Verification items for the finished model (mm, model axes). A direction names the side the tool comes from. Coordinates: 2 decimals unless noted, no trailing zeros. Order: outer loops, then holes, each group sorted by start corner. A loop starts at its lowest first (then second) coordinate and runs counter-clockwise, first axis right, second up. Notation, with made-up numbers: (-6.5, 60) -> (30.5, 60) arc R26 ccw to (30.5, 89) -> close; hole circle Ø1 at (74.5, -4). An arc over 180 degrees is marked (long way). Answer as CSV lines item,"result".
```python
from build123d import *

# Parameters (mm, degrees)
SZKIC1_R                    = 14
DODANIE_WYCI_GNI_CIE1_DEPTH = 4.5
SFAZOWANIE2_SIZE2           = 4.345599487
SFAZOWANIE2_SIZE            = 4.5
DODANIE_WYCI_GNI_CIE5_DEPTH = 12
WYTNIJ_WYCI_GNI_CIE2_DEPTH  = 8
SFAZOWANIE4_SIZE            = 4.5
SFAZOWANIE4_SIZE2           = 4.95
ZAOKR_GLENIE2_R             = 0.5
ZAOKR_GLENIE3_R             = 10.5
WYTNIJ_WYCI_GNI_CIE3_DEPTH  = 6


# Some blends are built 0.0001 mm under size
with BuildPart() as part:
    # Szkic1 → Dodanie-wyciągnięcie1 (new body)
    with BuildSketch(Plane.XY):
        Circle(SZKIC1_R)
    extrude(amount=DODANIE_WYCI_GNI_CIE1_DEPTH)

    # Sfazowanie2
    sfazowanie2_edges = [part.edges().sort_by_distance(p)[0] for p in [
        (-14, 0, 4.5),
    ]]
    sfazowanie2_side = [part.faces().sort_by_distance(p)[0] for p in [
        (-14, 0, 4.41308801),
    ]]
    chamfer(sfazowanie2_edges, length=SFAZOWANIE2_SIZE - 0.0001, length2=SFAZOWANIE2_SIZE2 - 0.0001, reference=sfazowanie2_side[0])  # a hair under: the kernel refuses the full size

    # Szkic2 → Dodanie-wyciągnięcie5 (add)
    with BuildSketch(Plane.XY.offset(4.5)):
        with BuildLine():
            Line((9.452124483, 1.965907434), (-0.429502914, 3.5))
            Line((-0.429502914, 3.5), (-8.99763576, 3.5))
            ThreePointArc((-8.99763576, 3.5), (-9.786966842, 0), (-8.99763576, -3.5))
            Line((-8.99763576, -3.5), (-0.429502914, -3.5))
            Line((-0.429502914, -3.5), (9.452124483, -1.965907434))
            ThreePointArc((9.452124483, -1.965907434), (9.654400513, 0), (9.452124483, 1.965907434))
        make_face()
    extrude(amount=DODANIE_WYCI_GNI_CIE5_DEPTH)

    # Szkic8 → Wytnij-wyciągnięcie2 (cut)
    with BuildSketch(Plane(origin=(0, 0, 0), x_dir=(-1, 0, 0), z_dir=(0, 0, -1))):
        with BuildLine():
            Line((-9.452124483, 1.965907434), (-13.654313406, 3.091880562))
            ThreePointArc((-13.654313406, 3.091880562), (-14.042737349, 0), (-13.654313406, -3.091880562))
            Line((-13.654313406, -3.091880562), (-9.452124483, -1.965907434))
            ThreePointArc((-9.452124483, -1.965907434), (-9.654400513, 0), (-9.452124483, 1.965907434))
        make_face()
    extrude(amount=-WYTNIJ_WYCI_GNI_CIE2_DEPTH, mode=Mode.SUBTRACT)

    # Sfazowanie4
    sfazowanie4_edges = [part.edges().sort_by_distance(p)[0] for p in [
        (9.654400513, 0, 16.5),
    ]]
    sfazowanie4_side = [part.faces().sort_by_distance(p)[0] for p in [
        (9.654400513, 0, 8.25),
    ]]
    chamfer(sfazowanie4_edges, length=SFAZOWANIE4_SIZE, length2=SFAZOWANIE4_SIZE2, reference=sfazowanie4_side[0])

    # Zaokrąglenie2
    zaokr_glenie2_edges = [part.edges().sort_by_distance(p)[0] for p in [
        (-9.786966842, 0, 16.5),
        (-4.713569337, -3.5, 16.5),
        (1.655695985, -3.17627922, 16.5),
        (-4.713569337, 3.5, 16.5),
        (1.655695985, 3.17627922, 16.5),
        (4.704400513, 0, 16.5),
        (6.663505686, 2.398832011, 14.338418901),
        (9.654400513, 0, 12),
        (6.663505686, -2.398832011, 14.338418901),
    ]]
    fillet(zaokr_glenie2_edges, radius=ZAOKR_GLENIE2_R)

    # Zaokrąglenie3
    # the kernel refuses this fillet: 10.5 mm, written as the material it takes off along each edge
    with BuildSketch(Plane(origin=(-1.239696749, -7, 16.5), x_dir=(0.15340925660527832, 0.9881627396273429, 0), z_dir=(0.9881627396273429, -0.15340925660527832, 0))) as zaokr_glenie3_piece_1:
        with BuildLine():
            CenterArc((10, -0.5), 0.5, 0, 90)
            Line((10.5, -0.5), (10.5, 0))
            Line((10.5, 0), (10, 0))
        make_face()
    revolve(axis=Axis((-1.239696749, -7, 16.5), (0, 0, 1)), revolution_arc=8.824549996, mode=Mode.SUBTRACT)
    with BuildSketch(Plane(origin=(-1.239696749, 7, 16.5), x_dir=(0, -1, 0), z_dir=(-1, 0, 0))) as zaokr_glenie3_piece_2:
        with BuildLine():
            CenterArc((10, -0.5), 0.5, 0, 90)
            Line((10.5, -0.5), (10.5, 0))
            Line((10.5, 0), (10, 0))
        make_face()
    revolve(axis=Axis((-1.239696749, 7, 16.5), (0, 0, 1)), revolution_arc=8.824549996, mode=Mode.SUBTRACT)
    with BuildSketch(Plane(origin=(-0.429502914, -3.5, 4.5), x_dir=(0.9881627396273429, 0.15340925660527846, 0), z_dir=(0, 0, 1))) as zaokr_glenie3_piece_3:
        with BuildLine():
            CenterArc((ZAOKR_GLENIE3_R * 0.0771613176062, ZAOKR_GLENIE3_R), ZAOKR_GLENIE3_R, 261.175450004, 8.824549996)
            Line((-ZAOKR_GLENIE3_R * 0.076247938999, ZAOKR_GLENIE3_R * 0.0118372603727), (0, 0))
            Line((0, 0), (ZAOKR_GLENIE3_R * 0.0771613176062, 0))
        make_face()
    extrude(amount=12, mode=Mode.SUBTRACT)
    with BuildSketch(Plane(origin=(-0.429502914, 3.5, 4.5), x_dir=(0.9881627396273429, -0.15340925660527815, 0), z_dir=(0, 0, 1))) as zaokr_glenie3_piece_4:
        with BuildLine():
            CenterArc((ZAOKR_GLENIE3_R * 0.0771613176062, -ZAOKR_GLENIE3_R), ZAOKR_GLENIE3_R, 90, 8.824549996)
            Line((-ZAOKR_GLENIE3_R * 0.076247938999, -ZAOKR_GLENIE3_R * 0.0118372603727), (0, 0))
            Line((0, 0), (ZAOKR_GLENIE3_R * 0.0771613176062, 0))
        make_face()
    extrude(amount=12, mode=Mode.SUBTRACT)

    # Szkic9 → Wytnij-wyciągnięcie3 (cut)
    with BuildSketch(Plane(origin=(0, 0, 0), x_dir=(-1, 0, 0), z_dir=(0, 0, -1))):
        with BuildLine():
            Line((1.17, -1.149217125), (-1.17, -1.149217125))
            ThreePointArc((-1.17, -1.149217125), (0, 1.64), (1.17, -1.149217125))
        make_face()
    extrude(amount=-WYTNIJ_WYCI_GNI_CIE3_DEPTH, mode=Mode.SUBTRACT)


solid = part.part
```
Item 1: Section check B-B, the plane z = 3.5. Record the boundary of the cut face in (x, y), plus the area to 3 significant figures.
Answer list:
outline,"(9.45, -1.97) arc R9.65 ccw to (9.45, 1.97) -> (10.39, 2.22) arc R10.62 ccw (long way) to (10.39, -2.22) -> close; hole (-1.17, -1.15) -> (1.17, -1.15) arc R1.64 ccw (long way) to start"
area,"343 mm2"
Item 2: Depth check by flat-ended pin: pin 1 Ø8.5 at (x, z) = (-5.5, 9.5) entering from +Y; pin 2 Ø1 at (y, z) = (4.5, 12.5) entering from -X; pin 3 Ø3 at (x, y) = (-9, -8) entering from +Z; pin 4 Ø2.5 at (x, y) = (1, -5.5) entering from +Z. Enter the tip coordinate at first touch or a pass-through.
Answer list:
pin 1,"y = 3.5"
pin 2,"through"
pin 3,"z = 3.58"
pin 4,"z = 4.5"
Item 3: Thickness scan on line 1 (Z direction, x = -2, y = -8); line 2 (X direction, y = 0, z = 1.2); line 3 (Y direction, x = 0, z = 1.45). Record the ranges inside material, lowest first.
Answer list:
line 1,"0 to 4.5"
line 2,"-12.84 to -1.64, 1.64 to 9.65"
line 3,"-12.6 to -1.15, 1.64 to 12.6"
Item 4: Release check for a two-part mould opening along Y. For faces 1 (the flat face through (0, 0, 6)), 2 (the cylindrical face through (-0.421, 3.468, 10.17)), 3 (the flat face through (4.85, -2.68, 10.17)) record: +Y half, -Y half, draft (parallel to the pull), parting line (faces both ways), or undercut.
Answer list:
face 1,"undercut"
face 2,"+Y half"
face 3,"-Y half"
Item 5: Tool access check on faces 4 (the cylindrical face through (-9.787, 0.051, 10.17)), 5 (the cylindrical face through (-0.44, -3.47, 10.17)), 6 (the flat face through (-5, 3.5, 10)), 7 (the flat face through (11.057, 2.396, 1.719)). Record the directions out of +Z, -Z, +X, -X, +Y, -Y that give a thin tool (end or side, any length) a straight path to the whole face; none if there is none.
Answer list:
face 4,"+Z, -X"
face 5,"+Z, +X, -Y"
face 6,"+Z, +X, -X, +Y"
face 7,"+Z, -Z, +X"
Item 6: Section check A-A, the plane z = 9.25. Record the boundary of the cut face in (x, y), plus the area to 3 significant figures.
Answer list:
outline,"(-9, -3.5) -> (-1.24, -3.5) arc R10.5 ccw to (0.37, -3.38) -> (9.45, -1.97) arc R9.65 ccw to (9.45, 1.97) -> (0.37, 3.38) arc R10.5 ccw to (-1.24, 3.5) -> (-9, 3.5) arc R8.15 ccw to start"
area,"118 mm2"
